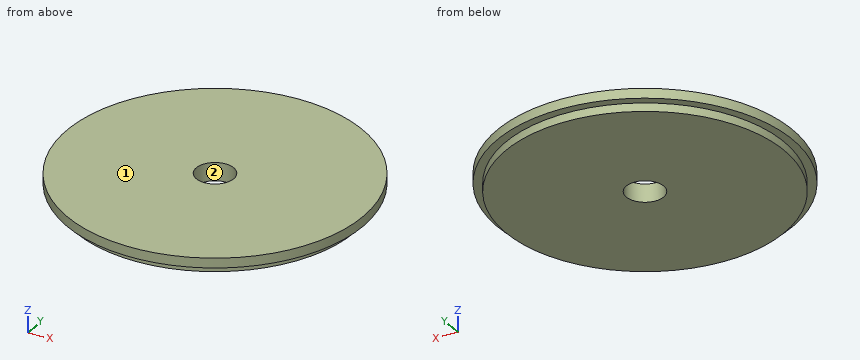
from build123d import *

# Parameters (mm, degrees)
F0_R     = 13.5255
F1_DEPTH = 0.889
F2_R     = 12.7635
F3_DEPTH = 1.651
F4_R     = 1.7145
F5_DEPTH = 1.652


with BuildPart() as f1:
    # F0 (on Top) → F1 (new body)
    with BuildSketch(Plane.XY):
        Circle(F0_R)
    extrude(amount=-F1_DEPTH)

    # F2 (on face) → F3 (join)
    with BuildSketch(Plane.XY):
        Circle(F2_R)
    extrude(amount=-F3_DEPTH)

    # F4 (on face) → F5 (cut, through all)
    with BuildSketch(Plane.XY):
        Circle(F4_R)
    extrude(amount=-F5_DEPTH, mode=Mode.SUBTRACT)


solid = f1.part
Here's how the part is built. I have some questions about the finished solid (model axes, mm). Face numbers are marked on the shaded views. Coordinates: 2 decimals unless noted, no trailing zeros. Order: outer loops, then holes, each group sorted by start corner. A loop starts at its lowest first (then second) coordinate and runs counter-clockwise, first axis right, second up.
Item 1: If we section it at A-A on x = 0: List the corners of the cut face in (y, z) for me, plus the area to 3 significant figures.
Result sheet:
outline: (-13.53, -0.89) - (-12.76, -0.89) - (-12.76, -1.65) - (-1.71, -1.65) - (-1.71, 0) - (-13.53, 0) - close; (1.71, -1.65) - (12.76, -1.65) - (12.76, -0.89) - (13.53, -0.89) - (13.53, 0) - (1.71, 0) - close
area: 37.8 mm2
Item 2: If we mould it in two halves opening along Y, with no side actions, what happens to the marked faces 1 and 2? For each: +Y half, -Y half, draft (parallel to the pull), parting line (faces both ways), or undercut.
Result sheet:
face 1: draft
face 2: undercut
Item 3: I need wall thicknesses on line 1 (Y direction, x = 0, z = -0.6); line 2 (Z direction, x = 6.25, y = 11.5); line 3 (X direction, y = -1.25, z = -0.8). Which ranges of each line are inside material? Lowest first, please.
Result sheet:
line 1: y = -13.53 to -1.71, 1.71 to 13.53
line 2: z = -0.89 to 0
line 3: x = -13.47 to -1.17, 1.17 to 13.47
Item 4: If we section it at D-D on y = 11.25: List the corners of the cut face in (x, z) for me, plus the area to 3 significant figures.
Result sheet:
outline: (-7.51, -0.89) - (-6.03, -0.89) - (-6.03, -1.65) - (6.03, -1.65) - (6.03, -0.89) - (7.51, -0.89) - (7.51, 0) - (-7.51, 0) - close
area: 22.5 mm2
Item 5: If we section it at C-C on z = -1.15: List the corners of the cut face in (x, y) for me.
Result sheet:
outline: circle Ø25.53 at (0, 0); hole circle Ø3.43 at (0, 0)
